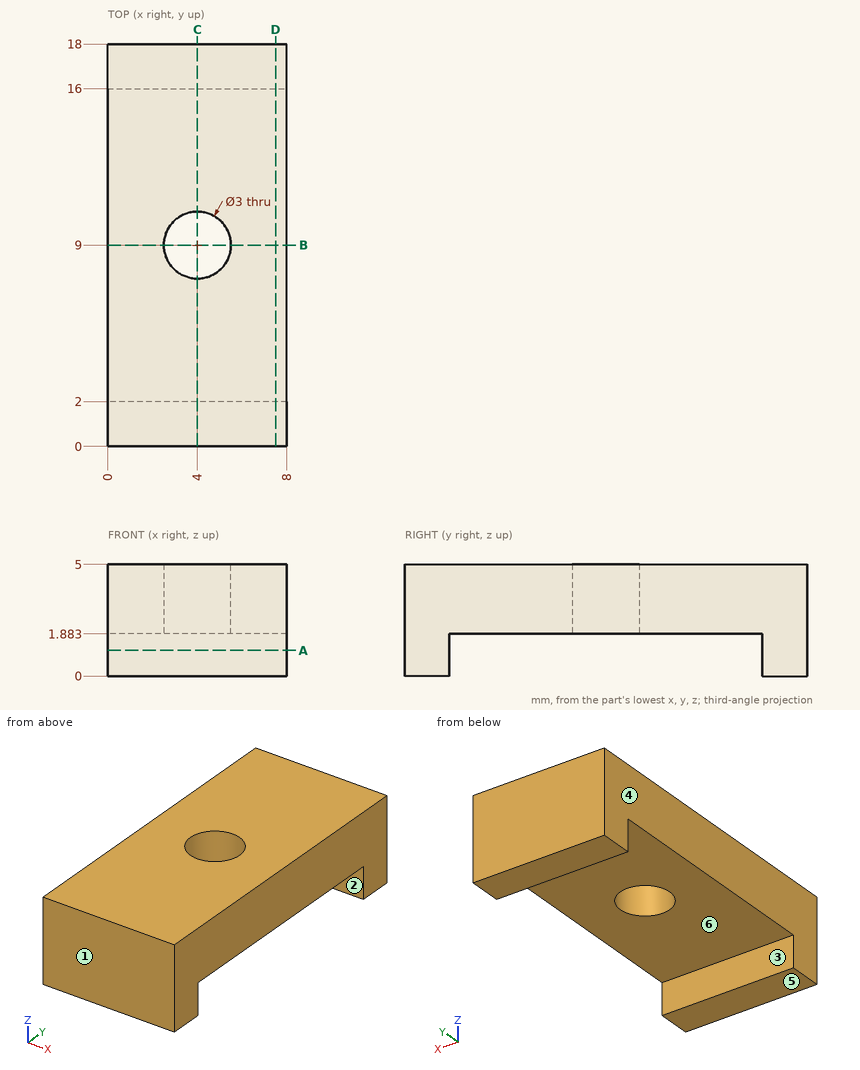
Drawing for the job (mm, zero at the part's lowest x, y, z). A direction names the side the tool comes from. Round coordinates to 2 decimals unless told otherwise and drop trailing zeros. Write each loop counter-clockwise with the first axis right and the second up, starting at its lowest first coordinate (ties: lowest second). Pieces come first, ordered by that corner, then holes. Notation, with made-up numbers: M 40,36.25 L 67,36.25 A30 ccw 67,73.25 Z; hole C -25.5,11.5 d10. An arc over 180 degrees is marked long. Answer in a Markdown table with one row per item.
1. Saw through at B-B (y = 9). List the corners of the cut face in (x, z).
Geometry check:
| item | result |
|---|---|
| outline | M 0,1.88 L 2.5,1.88 L 2.5,5 L 0,5 Z; M 5.5,1.88 L 8,1.88 L 8,5 L 5.5,5 Z |
2. Saw through at A-A (z = 1.15). List the corners of the cut face in (x, y).
Geometry check:
| item | result |
|---|---|
| outline | M 0,0 L 8,0 L 8,2 L 0,2 Z; M 0,16 L 8,16 L 8,18 L 0,18 Z |
3. Saw through at D-D (x = 7.5). List the corners of the cut face in (y, z).
Geometry check:
| item | result |
|---|---|
| outline | M 0,0 L 2,0 L 2,1.88 L 16,1.88 L 16,0 L 18,0 L 18,5 L 0,5 Z |
4. Probe L1, parallel to Y at x = 3.5, z = 1.85; L2, parallel to X at y = 9, z = 4.25; L3, parallel to Y at x = 4, z = 3.7. List the from-to ranges inside material, lowest first. Write a range as [from, to].
Geometry check:
| item | result |
|---|---|
| L1 | [0, 2], [16, 18] |
| L2 | [0, 2.5], [5.5, 8] |
| L3 | [0, 7.5], [10.5, 18] |
5. Mould opens along Y. For the marked faces 1, 2, 3 and 4 say: +Y half, -Y half, draft (parallel to the pull), parting line (faces both ways), or undercut.
Geometry check:
| item | result |
|---|---|
| face 1 | -Y half |
| face 2 | undercut |
| face 3 | undercut |
| face 4 | draft |
6. Saw through at C-C (x = 4). List the corners of the cut face in (y, z), and give its area (3 significant figures).
Geometry check:
| item | result |
|---|---|
| outline | M 0,0 L 2,0 L 2,1.88 L 7.5,1.88 L 7.5,5 L 0,5 Z; M 10.5,1.88 L 16,1.88 L 16,0 L 18,0 L 18,5 L 10.5,5 Z |
| area | 54.3 mm2 |
7. Flat gauge pins, fed straight in: P1, Ø2.5, axis at x = 4, y = 9, coming from the +Z side; P2, Ø2.5, axis at x = 2, y = 12.5, coming from the -Z side. Where does each tip first touch, or does it go through?
Geometry check:
| item | result |
|---|---|
| P1 | through |
| P2 | z = 1.88 |
8. Which spindle directions (+Z, -Z, +X, -X, +Y, -Y) get a long thin tool onto all of the face, cutting with end or side? Do the marked faces 5 and 6. Say none if no direction does.
Geometry check:
| item | result |
|---|---|
| face 5 | -Z, +X, -X, +Y, -Y |
| face 6 | -Z, +X, -X |
